Autodesk Inventor part; units mm, degrees
ref_plane "YZ Plane" through (0, 0, 0) normal (1, 0, 0) x (0, 1, 0)
ref_plane "XZ Plane" through (0, 0, 0) normal (0, 1, 0) x (-1, 0, 0)
ref_plane "XY Plane" through (0, 0, 0) normal (0, 0, 1) x (1, 0, 0)
sketch "Sketch1" plane through (0, 0, 0) normal (1, 0, 0) x (0, 1, 0)
  line L0 (0, 0) -> (0, 597.7382)
  line L1 (0, 0) -> (3.175, 0)
  line L2 (3.175, 0) -> (3.175, 594.5632)
  line L3 (3.175, 594.5632) -> (9.906, 594.5632)
  line L4 (9.906, 594.5632) -> (15.756, 595.9828)
  line L5 (0, 597.7382) -> (9.5263, 597.7382)
  line L6 (9.5263, 597.7382) -> (12.7824, 598.5283)
  line L7 (41.2921, 902.0052) -> (15.756, 595.9828)
  line L8 (12.7824, 598.5283) -> (38.1281, 902.2692)
  line L9 (38.1281, 902.2692) -> (41.2921, 902.0052)
  line L10 (41.2921, 902.0052) -> (44.4671, 901.7403)
  line L11 (44.4671, 901.7403) -> (18.7409, 593.44)
  line L12 (18.7409, 593.44) -> (10.2857, 591.3882)
  line L13 (10.2857, 591.3882) -> (6.35, 591.3882)
  line L14 (6.35, 591.3882) -> (6.35, 574.5988)
  line L15 (6.35, 574.5988) -> (3.175, 574.5988)
  line L16 (44.4671, 901.7403) -> (47.6311, 901.4763)
  line L17 (47.6311, 901.4763) -> (21.7146, 590.8944)
  line L18 (21.7146, 590.8944) -> (10.6654, 588.2132)
  line L19 (10.6654, 588.2132) -> (9.525, 588.2132)
  line L20 (9.525, 588.2132) -> (9.525, 432.9684)
  line L21 (9.525, 432.9684) -> (6.35, 432.9684)
  line L22 (6.35, 432.9684) -> (6.35, 574.5988)
  line L23 (32.5862, 759.3601) -> (35.7502, 759.0961)
  line L24 (47.6311, 901.4763) -> (50.7951, 901.2122)
  line L25 (50.7951, 901.2122) -> (24.6882, 588.3489)
  line L26 (24.6882, 588.3489) -> (13.2454, 585.5721)
  line L27 (13.2454, 585.5721) -> (12.7, 585.5721)
  line L28 (12.7, 585.5721) -> (12.7, 289.5351)
  line L29 (23.8692, 616.7159) -> (27.0332, 616.4519)
  line L30 (12.7, 289.5351) -> (9.525, 289.5351)
  line L31 (9.525, 289.5351) -> (9.525, 432.9684)
  line L32 (15.875, 582.9431) -> (20.5529, 584.0783)
  line L33 (15.875, 582.9431) -> (15.875, 573.3366)
  point P0 (14.5133, 592.4141)
  dimension "d0" = 594.5632
  dimension "d1" = 3.175
  dimension "d2" = 6.731
  dimension "d7" = 3.175
  dimension "d8" = 6.0198
  dimension "d9" = 166.36
  dimension "d10" = 3.175
  dimension "d11" = 108.41
  dimension "d12" = 3.175
  dimension "d13" = 307.086
  dimension "d18" = 3.175
  dimension "d20" = 307.1025
  dimension "d21" = 8.7006
  dimension "d22" = 3.175
  dimension "d23" = 3.175
  dimension "d24" = 3.9357
  dimension "d25" = 16.7894
  dimension "d28" = 3.175
  dimension "d29" = 3.186
  dimension "d30" = 3.175
  dimension "d32" = 3.175
  dimension "d33" = 3.175
  dimension "d34" = 142.875
  dimension "d35" = 168.7862
  dimension "d36" = 11.3698
  dimension "d37" = 1.1404
  dimension "d38" = 155.2448
  dimension "d41" = 3.175
  dimension "d42" = 3.175
  dimension "d43" = 3.175
  dimension "d44" = 142.875
  dimension "d45" = 296.037
  dimension "d46" = 28.2007
  dimension "d47" = 11.7749
  dimension "d48" = 0.5454
  dimension "d51" = 3.175
  dimension "d52" = 3.175
  dimension "d53" = 2.629
extrude "Extrusion4" add sketch "Sketch1" along normal blind 1000.125 contours L20 L19 L18 L17 L29 L25 L26 L27 L28 L30 L31
properties part number "Third_Shingle_Over_Intake_Vent_With_Length_39.375_Inches"
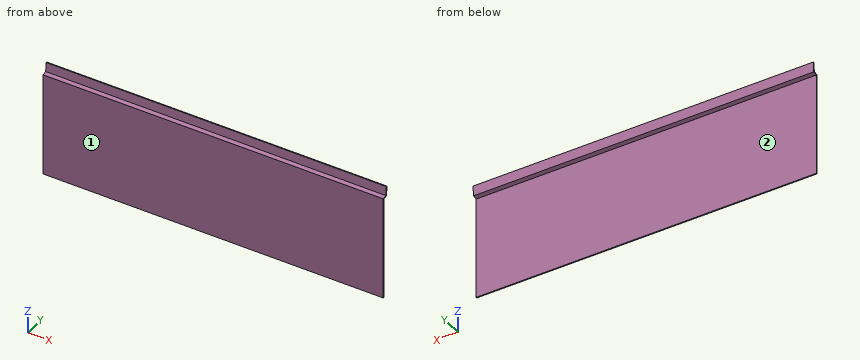
Design review of the part built by this model. Coordinates are the model's own, in mm. Face numbers are marked on the shaded views. A direction names the side the tool comes from. Give positions to 0.01 mm unless a question says otherwise; leave off trailing zeros. Order: outer loops, then holes, each group sorted by start corner. A loop starts at its lowest first (then second) coordinate and runs counter-clockwise, first axis right, second up. Notation, with made-up numbers: (53.25, 71.25) -> (84.25, 71.25) arc R18 ccw to (84.25, 90.25) -> close; hole circle Ø11 at (84.25, -22). An arc over 180 degrees is marked (long way). Write item = value, one per line. Start each with the question number.
(1) We need section B-B on z = 311.5. Write out the cut boundary in (x, y) (3 decimals), plus the area to 3 significant figures.
(2) We need section A-A on x = 123. Write out the cut boundary in (y, z) (3 decimals), plus the area to 3 significant figures.
(3) For pin 1 (6 mm diameter, centred on y = 13, z = 514.5, fed in from +X) (3 decimals); pin 2 (0.6 mm diameter, centred on x = 712.5, y = 10, fed in from +Z); pin 3 (3 mm diameter, centred on x = 490, y = 19.5, fed in from -Z); pin 4 (4 mm diameter, centred on x = 742.5, y = 19.5, fed in from +Z), all flat-tipped, find the tip position at first contact; note any pin that passes through.
(4) For the marked faces 1 and 2, list the 3-axis set-ups (+Z, -Z, +X, -X, +Y, -Y) from which the entire face can be reached by the end or side of a thin tool; tool diameter is ignored.
(5) We need section C-C on y = 17.5. Write out the cut boundary in (x, z) (3 decimals), plus the area to 3 significant figures.
(6) To check wall thickness, follow line 1 along Z through (x, y) = (102, 12); line 2 along Y through (x, z) = (648.5, 521.5) (3 decimals); line 3 along Z through (x, y) = (430, 24.5). State the ranges of each line that lie inside material, in increasing order.
Numbers:
q1.outline = (0, 9.525) -> (1000.125, 9.525) -> (1000.125, 12.7) -> (0, 12.7) -> close
q1.area = 3,180 mm^2
q2.outline = (9.525, 289.535) -> (12.7, 289.535) -> (12.7, 585.572) -> (13.245, 585.572) -> (24.688, 588.349) -> (27.033, 616.452) -> (23.869, 616.716) -> (21.715, 590.894) -> (10.665, 588.213) -> (9.525, 588.213) -> close
q2.area = 1,070 mm^2
q3.pin_1 = 1000.125
q3.pin_2 = 588.21
q3.pin_3 = 586.73
q3.pin_4 = 590.84
q4.face_1 = +Z, -Z, +X, -X, -Y
q4.face_2 = -Z, +X, -X, +Y
q5.outline = (0, 586.605) -> (1000.125, 586.605) -> (1000.125, 589.872) -> (0, 589.872) -> close
q5.area = 3,270 mm^2
q6.line_1 = 289.54 to 588.54
q6.line_2 = 9.525 to 12.7
q6.line_3 = 588.3 to 616.66
